Input: dimensioned drawing with shaded views. Units: mm. Origin: part minimum x, y, z. A direction names the side the tool comes from. Give positions to 0.01 mm unless a question says otherwise; leave off trailing zeros. Loops run counter-clockwise (first coordinate to the right, second up) from the corner with the lowest first, then second, coordinate; pieces in that order, holes last.
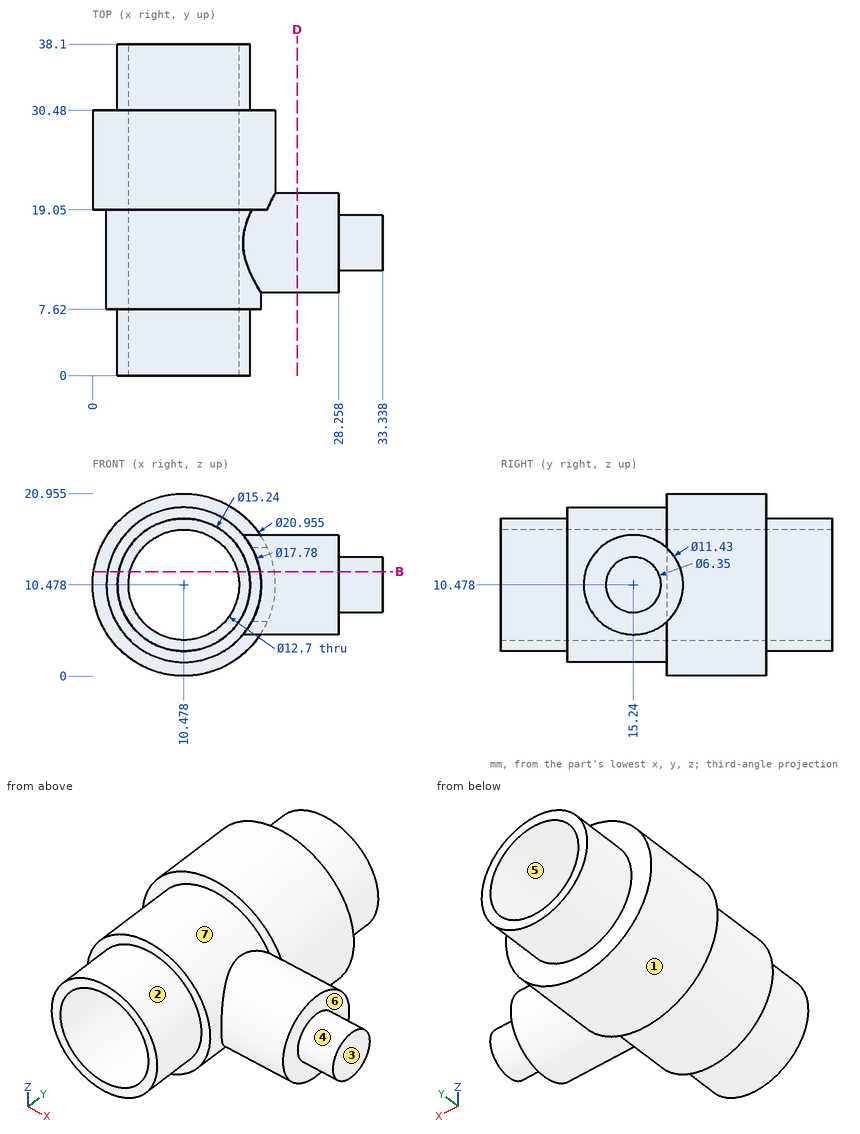
(1) First-contact query: pin 1 (4 mm diameter, centred on y = 9, z = 10.5, fed in from +X); pin 2 (4 mm diameter, centred on x = 25.5, z = 17, fed in from +Y) (1 decimal); pin 3 (4 mm diameter, centred on y = 29.5, z = 3.5, fed in from -X). Flat tips, straight axial feed; report the tip coordinate or a pass-through.
A:
pin 1: stops at x = 28.26
pin 2: stops at y = 18.7
pin 3: stops at x = 1.26
(2) Mould query, pull axis X, two halves, no side actions, for the marked faces 5, 6 and 7. Classes: pulls with the +X half, pulls with the -X half, needs draft (parallel to the pull), parting line crosses it, or undercut.
A:
face 5: undercut
face 6: pulls with the +X half
face 7: parting line crosses it
(3) Ray query, line 1 along Z through (x, y) = (15, 13) (1 decimal); line 2 along X through (y, z) = (6, 12) (1 decimal); line 3 along X through (y, z) = (11.5, 7.75) (1 decimal). Return the intervals inside material, ascending.
A:
line 1: z = 2.8 to 6, 14.9 to 18.1
line 2: x = 3 to 4.3, 16.6 to 17.9
line 3: x = 2 to 4.7, 16.2 to 28.3
(4) Reachability of the marked faces 1, 2, 3 and 4 from +Z, -Z, +X, -X, +Y, -Y: full face, straight path, thin tool, end or side. Return the list, or none.
A:
face 1: +Y
face 2: -Y
face 3: +Z, -Z, +X, +Y, -Y
face 4: +X
(5) Section D-D, the plane x = 23.5. Return the cut outline in (y, z) (1 decimal).
A:
outline: circle Ø11.4 at (15.2, 10.5)
(6) Section B-B, the plane z = 12. Return the cut outline in (x, y), then the cut area to 3 significant figures.
A:
outline: (0.11, 19.05) - (1.72, 19.05) - (1.72, 7.62) - (3.01, 7.62) - (3.01, 0) - (4.31, 0) - (4.31, 38.1) - (3.01, 38.1) - (3.01, 30.48) - (0.11, 30.48) - close; (16.64, 0) - (17.94, 0) - (17.94, 7.62) - (19.24, 7.62) - (19.24, 9.73) - (28.26, 9.73) - (28.26, 12.45) - (33.34, 12.45) - (33.34, 18.03) - (28.26, 18.03) - (28.26, 20.75) - (20.84, 20.75) - (20.84, 30.48) - (17.94, 30.48) - (17.94, 38.1) - (16.64, 38.1) - close
area: 320 mm2
